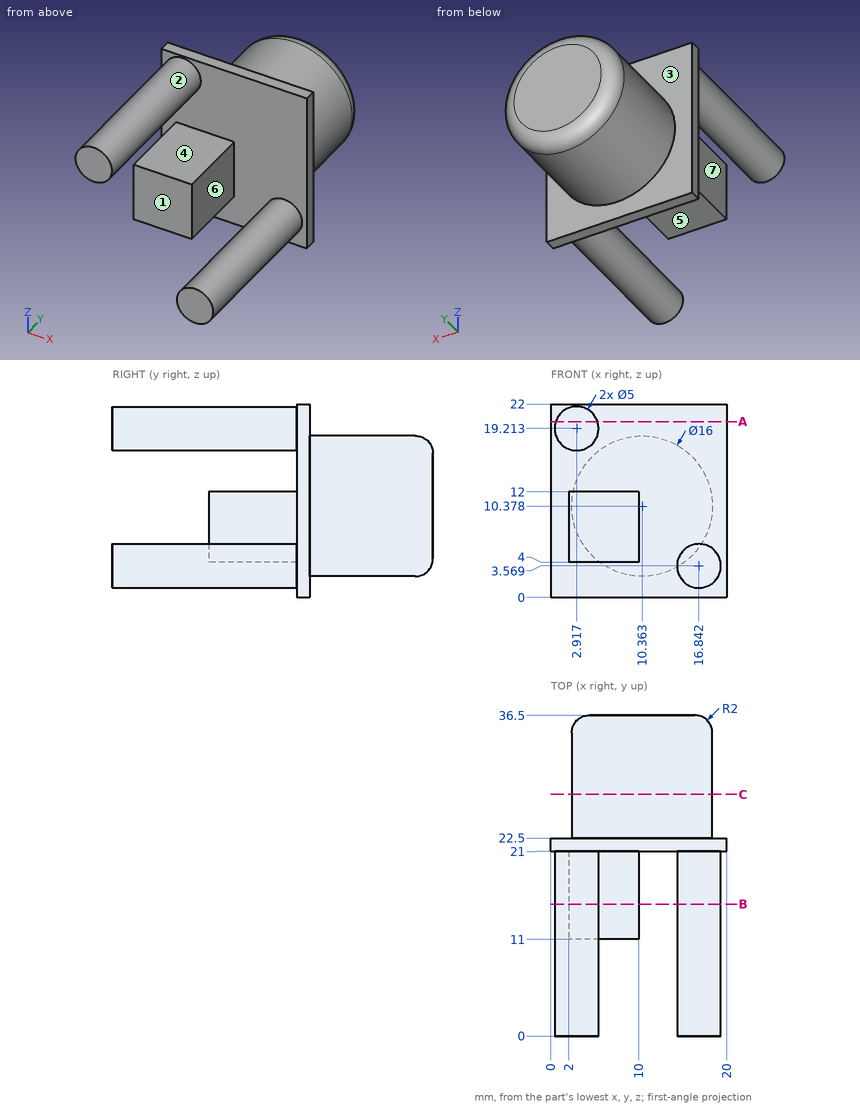
Part print with two shaded views. Sizes in mm from the minimum x, y, z corner. A direction names the side the tool comes from. Coordinates: 2 decimals unless noted, no trailing zeros. Order: outer loops, then holes, each group sorted by start corner. A loop starts at its lowest first (then second) coordinate and runs counter-clockwise, first axis right, second up. Notation, with made-up numbers: M -1.75,-27.5 L 24.25,-27.5 A13 ccw 24.25,-2.5 Z; hole C 65.25,33 d1. An arc over 180 degrees is marked long. Use a Markdown table: item, result.
(1) Pull direction X, two halves, no side cores. Call the marked faces 5, 6 and 7: released by +X, released by -X, zero draft, split by the parting line, or undercut.
A:
| item | result |
|---|---|
| face 5 | zero draft |
| face 6 | undercut |
| face 7 | released by -X |
(2) Cut at C-C on y = 27.5. Write the cut outline in (x, z).
A:
| item | result |
|---|---|
| outline | C 10.36,10.38 d16 |
(3) Cut at A-A on z = 20. Write the cut outline in (x, y).
A:
| item | result |
|---|---|
| outline | M 0,21 L 0.54,21 L 0.54,0 L 5.29,0 L 5.29,21 L 20,21 L 20,22.5 L 0,22.5 Z |
(4) Tool access for the marked faces 1, 2, 3 and 4: list every direction of +Z, -Z, +X, -X, +Y, -Y with a clear straight run to the whole face (end or side of a thin tool).
A:
| item | result |
|---|---|
| face 1 | -Z, -X, -Y |
| face 2 | -Y |
| face 3 | +Y |
| face 4 | +X, -X, -Y |
(5) Flat gauge pins, fed straight in: pin 1 (1 mm diameter, centred on x = 5, y = 29, fed in from +Z); pin 2 (8 mm diameter, centred on x = 15, z = 18, fed in from -Y); pin 3 (9 mm diameter, centred on x = 7.5, z = 7.5, fed in from -Y). Where does each tip first touch, or does it go through?
A:
| item | result |
|---|---|
| pin 1 | stops at z = 16.73 |
| pin 2 | stops at y = 21 |
| pin 3 | stops at y = 11 |
(6) Probe L1, parallel to Y at x = 9.75, z = 19.5; L2, parallel to Y at x = 5, z = 20; L3, parallel to X at y = 13.5, z = 8. List the from-to ranges inside material, lowest first.
A:
| item | result |
|---|---|
| L1 | y = 21 to 22.5 |
| L2 | y = 0 to 22.5 |
| L3 | x = 2 to 10 |
(7) Cut at B-B on y = 15. Write the cut outline in (x, z).
A:
| item | result |
|---|---|
| outline | C 2.92,19.21 d5; M 2,4 L 10,4 L 10,12 L 2,12 Z; C 16.84,3.57 d5 |
